Geometry check sheet. Reference: the model listing, model coordinates, mm. Face numbers are marked on the shaded views. Give positions to 0.01 mm unless a question says otherwise; leave off trailing zeros. Write each loop counter-clockwise with the first axis right and the second up, starting at its lowest first coordinate (ties: lowest second). Pieces come first, ordered by that corner, then holes. Notation, with made-up numbers: (39, 5.5) - (58, 5.5) arc R27 cw to (58, 28.5) - close; hole circle Ø10 at (24.25, 62.5). An arc over 180 degrees is marked (long way). Use a Markdown table: item, result.
```python
from build123d import *

# Parameters (mm, degrees)
SKETCH1_R           = 4
BOSS_EXTRUDE7_DEPTH = 1
BOSS_EXTRUDE8_START = 1
SKETCH1_4_R         = 4
BOSS_EXTRUDE8_DEPTH = 2.9


with BuildPart() as part:
    # Sketch1 → Boss-Extrude7 (new body)
    with BuildSketch(Plane(origin=(0, 0, 0), x_dir=(1, 0, 0), z_dir=(0, 1, 0))):
        with Locations(Location((0, 0, 0), (0, 0, 270))):
            Circle(SKETCH1_R)
    extrude(amount=BOSS_EXTRUDE7_DEPTH)

    # Sketch1<4> → Boss-Extrude8 (add)
    with BuildSketch(Plane(origin=(0, 0, 0), x_dir=(1, 0, 0), z_dir=(0, 1, 0)).offset(BOSS_EXTRUDE8_START)):
        with Locations(Location((0, 0, 0), (0, 0, 270))):
            Circle(SKETCH1_4_R)
        with BuildLine():
            Line((-0.34, 2.628098172), (0, 2.17))
            Line((0, 2.17), (0.3473, 2.627143451))
            ThreePointArc((0.3473, 2.627143451), (0.349543667, 2.62684587), (0.351787078, 2.626546373))
            Line((0.351787078, 2.626546373), (0.561637328, 2.096059043))
            Line((0.561637328, 2.096059043), (1.015420799, 2.447737854))
            ThreePointArc((1.015420799, 2.447737854), (1.017510995, 2.44686971), (1.019600449, 2.44599978))
            Line((1.019600449, 2.44599978), (1.085, 1.879275126))
            Line((1.085, 1.879275126), (1.614342348, 2.101522968))
            ThreePointArc((1.614342348, 2.101522968), (1.61613663, 2.100143422), (1.617929733, 2.098762344))
            Line((1.617929733, 2.098762344), (1.534421715, 1.534421715))
            Line((1.534421715, 1.534421715), (2.103249134, 1.612092764))
            ThreePointArc((2.103249134, 1.612092764), (2.104625225, 1.610295831), (2.10599978, 1.608497723))
            Line((2.10599978, 1.608497723), (1.879275126, 1.085))
            Line((1.879275126, 1.085), (2.448822968, 1.012801103))
            ThreePointArc((2.448822968, 1.012801103), (2.449687089, 1.01070924), (2.450549423, 1.00861664))
            Line((2.450549423, 1.00861664), (2.096059043, 0.561637328))
            Line((2.096059043, 0.561637328), (2.627513563, 0.34448872))
            ThreePointArc((2.627513563, 0.34448872), (2.627806826, 0.342244485), (2.628098172, 0.34))
            Line((2.628098172, 0.34), (2.17, 0))
            Line((2.17, 0), (2.627143451, -0.3473))
            ThreePointArc((2.627143451, -0.3473), (2.62684587, -0.349543667), (2.626546373, -0.351787078))
            Line((2.626546373, -0.351787078), (2.096059043, -0.561637328))
            Line((2.096059043, -0.561637328), (2.447737854, -1.015420799))
            ThreePointArc((2.447737854, -1.015420799), (2.44686971, -1.017510995), (2.44599978, -1.019600449))
            Line((2.44599978, -1.019600449), (1.879275126, -1.085))
            Line((1.879275126, -1.085), (2.101522968, -1.614342348))
            ThreePointArc((2.101522968, -1.614342348), (2.100143422, -1.61613663), (2.098762344, -1.617929733))
            Line((2.098762344, -1.617929733), (1.534421715, -1.534421715))
            Line((1.534421715, -1.534421715), (1.612092764, -2.103249134))
            ThreePointArc((1.612092764, -2.103249134), (1.610295831, -2.104625225), (1.608497723, -2.10599978))
            Line((1.608497723, -2.10599978), (1.085, -1.879275126))
            Line((1.085, -1.879275126), (1.012801103, -2.448822968))
            ThreePointArc((1.012801103, -2.448822968), (1.01070924, -2.449687089), (1.00861664, -2.450549423))
            Line((1.00861664, -2.450549423), (0.561637328, -2.096059043))
            Line((0.561637328, -2.096059043), (0.34448872, -2.627513563))
            ThreePointArc((0.34448872, -2.627513563), (0.342244485, -2.627806826), (0.34, -2.628098172))
            Line((0.34, -2.628098172), (0, -2.17))
            Line((0, -2.17), (-0.3473, -2.627143451))
            ThreePointArc((-0.3473, -2.627143451), (-0.349543667, -2.62684587), (-0.351787078, -2.626546373))
            Line((-0.351787078, -2.626546373), (-0.561637328, -2.096059043))
            Line((-0.561637328, -2.096059043), (-1.015420799, -2.447737854))
            ThreePointArc((-1.015420799, -2.447737854), (-1.017510995, -2.44686971), (-1.019600449, -2.44599978))
            Line((-1.019600449, -2.44599978), (-1.085, -1.879275126))
            Line((-1.085, -1.879275126), (-1.614342348, -2.101522968))
            ThreePointArc((-1.614342348, -2.101522968), (-1.61613663, -2.100143422), (-1.617929733, -2.098762344))
            Line((-1.617929733, -2.098762344), (-1.534421715, -1.534421715))
            Line((-1.534421715, -1.534421715), (-2.103249134, -1.612092764))
            ThreePointArc((-2.103249134, -1.612092764), (-2.104625225, -1.610295831), (-2.10599978, -1.608497723))
            Line((-2.10599978, -1.608497723), (-1.879275126, -1.085))
            Line((-1.879275126, -1.085), (-2.448822968, -1.012801103))
            ThreePointArc((-2.448822968, -1.012801103), (-2.449687089, -1.01070924), (-2.450549423, -1.00861664))
            Line((-2.450549423, -1.00861664), (-2.096059043, -0.561637328))
            Line((-2.096059043, -0.561637328), (-2.627513563, -0.34448872))
            ThreePointArc((-2.627513563, -0.34448872), (-2.627806826, -0.342244485), (-2.628098172, -0.34))
            Line((-2.628098172, -0.34), (-2.17, 0))
            Line((-2.17, 0), (-2.627143451, 0.3473))
            ThreePointArc((-2.627143451, 0.3473), (-2.62684587, 0.349543667), (-2.626546373, 0.351787078))
            Line((-2.626546373, 0.351787078), (-2.096059043, 0.561637328))
            Line((-2.096059043, 0.561637328), (-2.447737854, 1.015420799))
            ThreePointArc((-2.447737854, 1.015420799), (-2.44686971, 1.017510995), (-2.44599978, 1.019600449))
            Line((-2.44599978, 1.019600449), (-1.879275126, 1.085))
            Line((-1.879275126, 1.085), (-2.101522968, 1.614342348))
            ThreePointArc((-2.101522968, 1.614342348), (-2.100143422, 1.61613663), (-2.098762344, 1.617929733))
            Line((-2.098762344, 1.617929733), (-1.534421715, 1.534421715))
            Line((-1.534421715, 1.534421715), (-1.612092764, 2.103249134))
            ThreePointArc((-1.612092764, 2.103249134), (-1.610295831, 2.104625225), (-1.608497723, 2.10599978))
            Line((-1.608497723, 2.10599978), (-1.085, 1.879275126))
            Line((-1.085, 1.879275126), (-1.012801103, 2.448822968))
            ThreePointArc((-1.012801103, 2.448822968), (-1.01070924, 2.449687089), (-1.00861664, 2.450549423))
            Line((-1.00861664, 2.450549423), (-0.561637328, 2.096059043))
            Line((-0.561637328, 2.096059043), (-0.34448872, 2.627513563))
            ThreePointArc((-0.34448872, 2.627513563), (-0.342244485, 2.627806826), (-0.34, 2.628098172))
        make_face(mode=Mode.SUBTRACT)
    extrude(amount=BOSS_EXTRUDE8_DEPTH)


solid = part.part
```
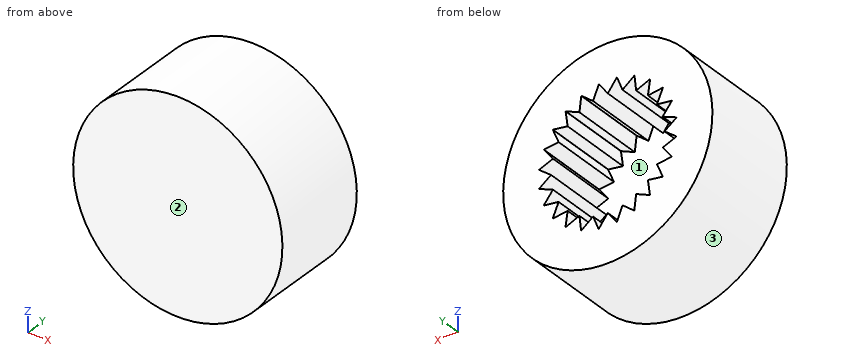
1) Section check A-A on z = 0.75. Record the boundary of the cut face in (x, y).
Working result:
| item | result |
|---|---|
| outline | (-3.93, 0) - (3.93, 0) - (3.93, 3.9) - (2.24, 3.9) - (2.24, 1) - (-2.25, 1) - (-2.25, 3.9) - (-3.93, 3.9) - close |
2) Section check B-B on x = -3. Record the boundary of the cut face in (y, z), then the cut area to 3 significant figures.
Working result:
| item | result |
|---|---|
| outline | (0, -2.65) - (3.9, -2.65) - (3.9, 2.65) - (0, 2.65) - close |
| area | 20.6 mm² |
3) Depth check by flat-ended pin: P1, Ø2, axis at x = 2.5, y = 3, coming from the -Z side. Enter the tip coordinate at first touch or a pass-through.
Working result:
| item | result |
|---|---|
| P1 | stops at z = -3.71 |
4) Mould release check, pull along X, two halves, no side actions. Record for the marked faces 1, 2 and 3: pulls with the +X half, pulls with the -X half, needs draft (parallel to the pull), parting line crosses it, or undercut.
Working result:
| item | result |
|---|---|
| face 1 | undercut |
| face 2 | needs draft |
| face 3 | parting line crosses it |
5) Section check C-C on z = 3. Record the boundary of the cut face in (x, y).
Working result:
| item | result |
|---|---|
| outline | (-2.65, 0) - (2.65, 0) - (2.65, 3.9) - (-2.65, 3.9) - close |
6) Material ranges on L1, parallel to Y at x = 2, z = -0.75; L2, parallel to Z at x = 2, y = 2.6; L3, parallel to Z at x = -0.75, y = 1.1, recorded low to high. Write a range as from..to.
Working result:
| item | result |
|---|---|
| L1 | y = 0..1 |
| L2 | z = -3.46..-1.6, -1.36..-1.07, 1.07..1.37, 1.6..3.46 |
| L3 | z = -3.93..-2.25, 2.24..3.93 |
